from build123d import *

# Parameters (mm, degrees)
BASPROSKE_W      = 13
BASPROSKE_H      = 15
TOOTHCUT_DEPTH   = 25.879710609
TEETHCUTS_COUNT  = 13
TEETHCUTS_ANGLE  = 332.307692308
HUBNEAONESKE_R   = 6
HUBNEARONE_DEPTH = 4.0000508
BORSKE_R         = 5
BORE_DEPTH       = 17.0000508
SCALE1_SCALE     = 0.317565217


with BuildPart() as part:
    # BasProSke → Base-Revolve (revolve)
    with BuildSketch(Plane(origin=(0, 0, 0), x_dir=(1, 0, 0), z_dir=(0, 1, 0)), mode=Mode.PRIVATE) as base_revolve_sk:
        with Locations((6.5, 7.5)):
            Rectangle(BASPROSKE_W, BASPROSKE_H)
    revolve(base_revolve_sk.sketch.rotate(Axis((-10, 0, 0), (1, 0, 0)), 180), axis=Axis((-10, 0, 0), (1, 0, 0)))

    # TooCutSke → ToothCut (cut, through all)
    with BuildSketch(Plane(origin=(0, 0, 0), x_dir=(0, 0, -1), z_dir=(1, 0, 0))):
        with BuildLine():
            ThreePointArc((1.088245291, 10.442448141), (0, 10.499), (-1.088245291, 10.442448141))
            ThreePointArc((-1.088245291, 10.442448141), (-1.646045958, 12.816546547), (-3.224884568, 14.675243258))
            ThreePointArc((-3.224884568, 14.675243258), (0, 15.0254), (3.224884568, 14.675243258))
            ThreePointArc((3.224884568, 14.675243258), (1.646045958, 12.816546547), (1.088245291, 10.442448141))
        make_face()
    toothcut = extrude(amount=TOOTHCUT_DEPTH, mode=Mode.SUBTRACT)

    # TeethCuts: ToothCut ×13 about axis
    teethcuts_axis = Axis((-10, 0, 0), (1, 0, 0))
    for i in range(1, TEETHCUTS_COUNT):
        add(toothcut.rotate(teethcuts_axis, i * TEETHCUTS_ANGLE / (TEETHCUTS_COUNT - 1)), mode=Mode.SUBTRACT)

    # HubNeaOneSke → HubNearOne (add)
    with BuildSketch(Plane.ZY):
        with Locations(Location((0, 0, 0), (0, 0, 180))):
            Circle(HUBNEAONESKE_R)
    extrude(amount=HUBNEARONE_DEPTH)

    # BorSke → Bore (cut, symmetric)
    with BuildSketch(Plane(origin=(0, 0, 0), x_dir=(0, 0, -1), z_dir=(1, 0, 0))):
        with Locations(Location((0, 0, 0), (0, 0, 180))):
            Circle(BORSKE_R)
    extrude(amount=BORE_DEPTH, both=True, mode=Mode.SUBTRACT)


with BuildPart() as part_1:
    # Scale1: scaled about (6.291140597, 0, 0)
    add(part.part.scale(SCALE1_SCALE).moved(Location((4.293293168, 0, 0))))


solid = part_1.part
Input: part model. Units: mm. Frame: model coordinates. A direction names the side the tool comes from. Coordinates: 2 decimals unless noted, no trailing zeros. Loops run counter-clockwise (first coordinate to the right, second up) from the corner with the lowest first, then second, coordinate; pieces in that order, holes last. Notation, with made-up numbers: (34, -27) -> (70, -27) arc R20 cw to (70, -6) -> close; hole circle Ø5 at (89, 85.25). An arc over 180 degrees is marked (long way). Write each question's results on one line, items separated by ' | '. Start each with the question number.
Q1. Section A-A, the plane z = 0. Return the cut outline in (x, y), plus the area to 3 significant figures.
Q2. Section B-B, the plane z = 2.75. Return the cut outline in (x, y).
Q3. Pull-direction query (Z, two-part tool) for faces 3 (the cylindrical face through (6.33, -4.06, 0.47)), 4 (the cylindrical face through (6.33, 3.85, 1.43)), 5 (the cylindrical face through (3.67, 1.86, 0.41)); classes: released by +Z, released by -Z, zero draft, split by the parting line, or undercut.
Q4. Ray query, line 1 (Y direction, x = 6.7, z = 0); line 2 (Y direction, x = 4.1, z = 0); line 3 (Y direction, x = 6.7, z = 3.5). Return the intervals inside material, ascending. Write a range as from..to.
Q5. Reachability of faces 1 (the cylindrical face through (6.329, -1.936, -3.624)), 2 (the cylindrical face through (6.329, -0.956, -3.975)) from +Z, -Z, +X, -X, +Y, -Y: full face, straight path, thin tool, end or side. Return the list, or none.
Q6. Pin query (flat end, axial travel): pin 1 (3 mm diameter, centred on x = 5.5, z = -2, fed in from -Y); pin 2 (1 mm diameter, centred on x = 4.5, y = 1, fed in from -Z); pin 3 (1.5 mm diameter, centred on x = 3.5, y = 1, fed in from -Z). Return the tip coordinate at first contact, or that it passes through.
Found:
1) outline: (3.02, -1.91) -> (4.29, -1.91) -> (4.29, -4.76) -> (8.42, -4.76) -> (8.42, -1.59) -> (3.02, -1.59) -> close; (3.02, 1.59) -> (8.42, 1.59) -> (8.42, 3.33) -> (4.29, 3.33) -> (4.29, 1.91) -> (3.02, 1.91) -> close | area: 21.1 mm2
2) outline: (4.29, -2.52) -> (8.42, -2.52) -> (8.42, 1.89) -> (4.29, 1.89) -> close; (4.29, 2.34) -> (8.42, 2.34) -> (8.42, 3.57) -> (4.29, 3.57) -> close
3) face 3: undercut | face 4: undercut | face 5: split by the parting line
4) line 1: -4.76..-1.59, 1.59..3.33 | line 2: -1.91..-1.59, 1.59..1.91 | line 3: -2.8..-1.81, -0.93..0.07, 0.79..1.85
5) face 1: -Z, +X, -X | face 2: +X, -X
6) pin 1: y = -4.28 | pin 2: z = -4.46 | pin 3: z = -1.89
